Check sheet for the modelled part. Datum: model origin and axes. Units: mm. Give positions to 0.01 mm unless a question says otherwise; leave off trailing zeros. Order: outer loops, then holes, each group sorted by start corner. A loop starts at its lowest first (then second) coordinate and runs counter-clockwise, first axis right, second up.
from build123d import *

# Parameters (mm, degrees)
SKETCH1_W           = 12.7
SKETCH1_H           = 12.7
BOSS_EXTRUDE1_DEPTH = 40
CUT_EXTRUDE1_DEPTH  = 43.445406112
SKETCH3_R           = 2.15
CUT_EXTRUDE2_DEPTH  = 43.445406112
SKETCH4_R           = 1.65
CUT_EXTRUDE3_DEPTH  = 43.445406112


with BuildPart() as part:
    # Sketch1 → Boss-Extrude1 (new, symmetric)
    with BuildSketch(Plane.XY):
        Rectangle(SKETCH1_W, SKETCH1_H)
    extrude(amount=BOSS_EXTRUDE1_DEPTH, both=True)

    # Sketch2 → Cut-Extrude1 (cut, through all)
    with BuildSketch(Plane(origin=(6.35, 0, 0), x_dir=(0, 0, -1), z_dir=(1, 0, 0))):
        with BuildLine():
            ThreePointArc((0, 2.375), (-10.776585121, 0), (0, -2.375))
            ThreePointArc((0, -2.375), (10.776585121, 0), (0, 2.375))
        make_face()
    extrude(amount=-CUT_EXTRUDE1_DEPTH, mode=Mode.SUBTRACT)

    # Sketch3 → Cut-Extrude2 (cut, through all)
    with BuildSketch(Plane(origin=(0, 6.35, 0), x_dir=(1, 0, 0), z_dir=(0, 1, 0))):
        with Locations(Location((0, 35, 0), (0, 0, 270))):
            Circle(SKETCH3_R)
        with Locations(Location((0, 20, 0), (0, 0, 270))):
            Circle(SKETCH3_R)
    extrude(amount=-CUT_EXTRUDE2_DEPTH, mode=Mode.SUBTRACT)

    # Sketch4 → Cut-Extrude3 (cut, through all)
    with BuildSketch(Plane(origin=(0, 6.35, 0), x_dir=(1, 0, 0), z_dir=(0, 1, 0))):
        with Locations(Location((0, -35, 0), (0, 0, 270))):
            Circle(SKETCH4_R)
        with Locations(Location((0, -20, 0), (0, 0, 270))):
            Circle(SKETCH4_R)
    extrude(amount=-CUT_EXTRUDE3_DEPTH, mode=Mode.SUBTRACT)


solid = part.part
1) Section check A-A, the plane y = 0. Record the cut outline in (x, z), then the cut area to 3 significant figures.
Recorded:
outline: (-6.35, -40) - (6.35, -40) - (6.35, -10.78) - (-6.35, -10.78) - close; (-6.35, 10.78) - (6.35, 10.78) - (6.35, 40) - (-6.35, 40) - close; hole circle Ø4.3 at (0, -35); hole circle Ø4.3 at (0, -20); hole circle Ø3.3 at (0, 20); hole circle Ø3.3 at (0, 35)
area: 696 mm2
2) Material ranges on L1, parallel to X at y = -3.5, z = -20; L2, parallel to Z at x = 2.75, y = 0; L3, parallel to Z at x = -3, y = 3.25, recorded low to high.
Recorded:
L1: x = -6.35 to -2.15, 2.15 to 6.35
L2: z = -40 to -10.78, 10.78 to 40
L3: z = -40 to -9.75, -0.5 to 0.5, 9.75 to 40
3) Section check C-C, the plane y = 4. Record the cut outline in (x, z), then the cut area to 3 significant figures.
Recorded:
outline: (-6.35, -40) - (6.35, -40) - (6.35, -9.12) - (-6.35, -9.12) - close; (-6.35, -1.14) - (6.35, -1.14) - (6.35, 1.14) - (-6.35, 1.14) - close; (-6.35, 9.12) - (6.35, 9.12) - (6.35, 40) - (-6.35, 40) - close; hole circle Ø4.3 at (0, -35); hole circle Ø4.3 at (0, -20); hole circle Ø3.3 at (0, 20); hole circle Ø3.3 at (0, 35)
area: 767 mm2
4) Depth check by flat-ended pin: pin 1 Ø5 at (x, z) = (0, -35) entering from +Y. Enter the tip coordinate at first touch or a pass-through.
Recorded:
pin 1: stops at y = 6.35
5) Draft check along Y on faces 1 (the face through (0, 6.35, 1)), 2 (the face through (-1, 0.09, 18.69)), 3 (the face through (0, -6.35, 1)), 4 (the face through (0.089, 0.214, 10.773)). Enter one of: +Y half, -Y half, draft (parallel to the pull), parting line (faces both ways), or undercut.
Recorded:
face 1: +Y half
face 2: draft
face 3: -Y half
face 4: undercut
6) Section check B-B, the plane z = 35. Record the cut outline in (x, y), then the cut area to 3 significant figures.
Recorded:
outline: (-6.35, -6.35) - (-1.65, -6.35) - (-1.65, 6.35) - (-6.35, 6.35) - close; (1.65, -6.35) - (6.35, -6.35) - (6.35, 6.35) - (1.65, 6.35) - close
area: 119 mm2
7) Section check D-D, the plane z = -35. Record the cut outline in (x, y), then the cut area to 3 significant figures.
Recorded:
outline: (-6.35, -6.35) - (-2.15, -6.35) - (-2.15, 6.35) - (-6.35, 6.35) - close; (2.15, -6.35) - (6.35, -6.35) - (6.35, 6.35) - (2.15, 6.35) - close
area: 107 mm2
